Verification items for the finished model (mm, model axes). A direction names the side the tool comes from. Coordinates: 2 decimals unless noted, no trailing zeros. Write each loop counter-clockwise with the first axis right and the second up, starting at its lowest first coordinate (ties: lowest second). Pieces come first, ordered by that corner, then holes. Notation, with made-up numbers: (44, 54) -> (91, 54) arc R22 cw to (91, 77) -> close; hole circle Ø6 at (87.5, 58.25). An arc over 180 degrees is marked (long way). Answer in a Markdown table with one row per item.
```python
from build123d import *

# Parameters (mm, degrees)
F0_W     = 650
F0_H     = 100
F1_DEPTH = 150
F2_W     = 250
F2_H     = 25
F3_DEPTH = 30
F5_DEPTH = 25
F6_R     = 5
F7_W     = 630
F7_H     = 130
F8_DEPTH = 90


with BuildPart() as f1:
    # F0 (on Front) → F1 (new body)
    with BuildSketch(Plane.XZ):
        Rectangle(F0_W, F0_H)
    extrude(amount=F1_DEPTH)

    # F2 (on face) → F3 (join)
    with BuildSketch(Plane.XZ.offset(150)):
        Rectangle(F2_W, F2_H)
    extrude(amount=F3_DEPTH)

    # F4 (on face) → F5 (cut)
    with BuildSketch(Plane.XY.offset(12.5)):
        Polygon((-120, -175), (120, -175), (120, -155), (120, -150), (-120, -150), (-120, -155), align=None)
    extrude(amount=-F5_DEPTH, mode=Mode.SUBTRACT)

    # F6
    f6_edges = [f1.edges().sort_by_distance(p)[0] for p in [
        (125, -150, 0),
        (-125, -150, 0),
        (-122.5, -150, 12.5),
        (-122.5, -150, -12.5),
        (-120, -150, 0),
        (120, -150, 0),
        (122.5, -150, -12.5),
        (122.5, -150, 12.5),
    ]]
    fillet(f6_edges, radius=F6_R)

    # F7 (on face) → F8 (cut)
    with BuildSketch(Plane.XY.offset(50)):
        with Locations((0, -75)):
            Rectangle(F7_W, F7_H)
    extrude(amount=-F8_DEPTH, mode=Mode.SUBTRACT)


solid = f1.part
```
1. Release check for a two-part mould opening along Y. For faces 1 (the face through (-5, 0, 1)), 2 (the face through (-19, -177, -12.5)), 3 (the face through (315, -76, 6)) record: released by +Y, released by -Y, zero draft, split by the parting line, or undercut.
Findings below:
| item | result |
|---|---|
| face 1 | released by +Y |
| face 2 | zero draft |
| face 3 | undercut |
2. Go/stop test with flat-tipped pins: pin 1 (12.5 mm diameter, centred on y = -161.5, z = -6, fed in from +X); pin 2 (1.5 mm diameter, centred on x = -171.5, z = -10.5, fed in from -Y); pin 3 (12.5 mm diameter, centred on y = -167, z = -1.5, fed in from -X). Record where each tip stops, or that it passes through.
Findings below:
| item | result |
|---|---|
| pin 1 | stops at x = 125 |
| pin 2 | stops at y = -150 |
| pin 3 | stops at x = -125 |
3. Access from +Z, -Z, +X, -X, +Y, -Y to the whole of each face (thin tool, end or side, straight path). Record for faces 4 (the face through (-2, -175, 0)), 5 (the face through (-125, -167, 0)), 6 (the face through (-4, -140, 6)), 7 (the face through (-19, -177, 12.5)), 8 (the face through (125, -167, 0)).
Findings below:
| item | result |
|---|---|
| face 4 | +Z, -Z |
| face 5 | +Z, -Z, -X, -Y |
| face 6 | +Z |
| face 7 | +Z, +X, -X, -Y |
| face 8 | +Z, -Z, +X, -Y |
4. Sectioned sample at A-A, the plane z = 1.5. Record the cut outline in (x, y), and give its area (3 significant figures).
Findings below:
| item | result |
|---|---|
| outline | (-325, -150) -> (-130, -150) arc R5 cw to (-125, -155) -> (-125, -180) -> (125, -180) -> (125, -155) arc R5 cw to (130, -150) -> (325, -150) -> (325, 0) -> (-325, 0) -> close; hole (-315, -140) -> (315, -140) -> (315, -10) -> (-315, -10) -> close; hole (-120, -175) -> (120, -175) -> (120, -155) arc R5 ccw to (115, -150) -> (-115, -150) arc R5 ccw to (-120, -155) -> close |
| area | 17,100 mm² |
5. Sectioned sample at D-D, the plane y = -86. Record the cut outline in (x, z).
Findings below:
| item | result |
|---|---|
| outline | (-325, -50) -> (325, -50) -> (325, 50) -> (315, 50) -> (315, -40) -> (-315, -40) -> (-315, 50) -> (-325, 50) -> close |
6. Sectioned sample at B-B, the plane x = -99.5. Record the cut outline in (y, z).
Findings below:
| item | result |
|---|---|
| outline | (-180, -12.5) -> (-175, -12.5) -> (-175, 12.5) -> (-180, 12.5) -> close; (-150, -50) -> (0, -50) -> (0, 50) -> (-10, 50) -> (-10, -40) -> (-140, -40) -> (-140, 50) -> (-150, 50) -> close |
7. Material ranges on probe 1 along Y at (x, z) = (77.5, -1); probe 2 along X at (y, z) = (-155, 1.5); probe 3 along X at (y, z) = (-60, -33), recorded low to high. Write a range as from..to.
Findings below:
| item | result |
|---|---|
| probe 1 | y = -180..-175, -150..-140, -10..0 |
| probe 2 | x = -125..-120, 120..125 |
| probe 3 | x = -325..-315, 315..325 |
8. Sectioned sample at C-C, the plane z = -28.5. Record the cut outline in (x, y), and give its area (3 significant figures).
Findings below:
| item | result |
|---|---|
| outline | (-325, -150) -> (325, -150) -> (325, 0) -> (-325, 0) -> close; hole (-315, -140) -> (315, -140) -> (315, -10) -> (-315, -10) -> close |
| area | 15,600 mm² |
